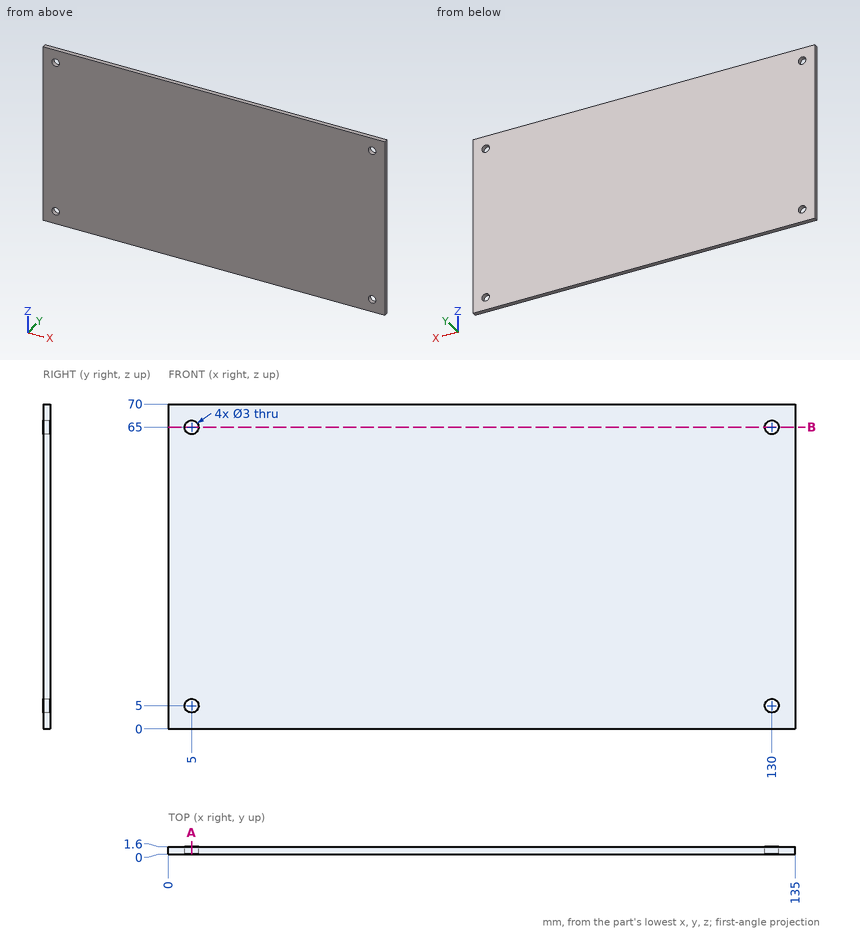
Job drawing, mm, ordinate dimensions from the low corner. One solid piece. Round coordinates to 2 decimals unless told otherwise and drop trailing zeros. Write each loop counter-clockwise with the first axis right and the second up, starting at its lowest first coordinate (ties: lowest second). Pieces come first, ordered by that corner, then holes. Notation, with made-up numbers: M 83,-1 L 124,-1 A14 ccw 124,21 Z; hole C -26,-22 d2. An arc over 180 degrees is marked long. Return JSON: item names as keys, results as strings. Group by question number.
(1) Saw through at A-A on x = 5. Write the cut outline in (y, z).
(2) Saw through at B-B on z = 65. Write the cut outline in (x, y).
(3) Drill centre lines: probe 1 along X at (y, z) = (0.95, 5); probe 2 along Z at (x, y) = (130, 1.05); probe 3 along X at (y, z) = (0.3, 4). Where is each one in solid material? Low to high.
Returned:
{
 "1": {"outline": "M 0,0 L 1.6,0 L 1.6,3.5 L 0,3.5 Z; M 0,6.5 L 1.6,6.5 L 1.6,63.5 L 0,63.5 Z; M 0,66.5 L 1.6,66.5 L 1.6,70 L 0,70 Z"},
 "2": {"outline": "M 0,0 L 3.5,0 L 3.5,1.6 L 0,1.6 Z; M 6.5,0 L 128.5,0 L 128.5,1.6 L 6.5,1.6 Z; M 131.5,0 L 135,0 L 135,1.6 L 131.5,1.6 Z"},
 "3": {"probe 1": "0 to 3.5, 6.5 to 128.5, 131.5 to 135", "probe 2": "0 to 3.5, 6.5 to 63.5, 66.5 to 70", "probe 3": "0 to 3.88, 6.12 to 128.88, 131.12 to 135"}
}
